Study the drawing (mm; zero at the part's minimum x, y, z) and answer. A direction names the side the tool comes from. Coordinates: 2 decimals unless noted, no trailing zeros. Order: outer loops, then holes, each group sorted by start corner. A loop starts at its lowest first (then second) coordinate and runs counter-clockwise, first axis right, second up. Notation, with made-up numbers: M 76.25,-11 L 121.25,-11 A24 cw 121.25,7 Z; hole C 48.25,42 d11. An arc over 180 degrees is marked long. Use a Markdown table: item, result. Add a question column.
1) Find section B-B on z = 51.5. Write down the section's boundary in (x, y).
2) Find section A-A on y = 12. Write down the section's boundary in (x, z).
3) Find section D-D on x = 88. Write down the section's boundary in (y, z), plus the area to 3 significant figures.
4) The mould has two halves that part along Y. Classify the marked faces 3, 4 and 5: released by +Y, released by -Y, zero draft, split by the parting line, or undercut.
5) Find section C-C on x = 17. Write down the section's boundary in (y, z).
6) Each of these flat-tipped pins is pushed along its axis until it touches: pin 1 Ø2.5 at (x, y) = (66, 45.5) entering from +Z; pin 2 Ø12.5 at (x, y) = (75, 20.5) entering from +Z; pin 3 Ø3.5 at (x, y) = (77.5, 2) entering from +Z. Where does it stop, or does it pass through?
7) Find the intervals of material crossed by probe 1 along Y at (x, z) = (119, 72); probe 2 along X at (y, z) = (34, 51.5); probe 3 along Y at (x, z) = (10, 19), in increasing order. Write a range as [from, to].
8) For the marked faces 1 and 2, determine the directions among +Z, -Z, +X, -X, +Y, -Y from which every point of the face is accessible in a straight line to the end or side of a thin tool.
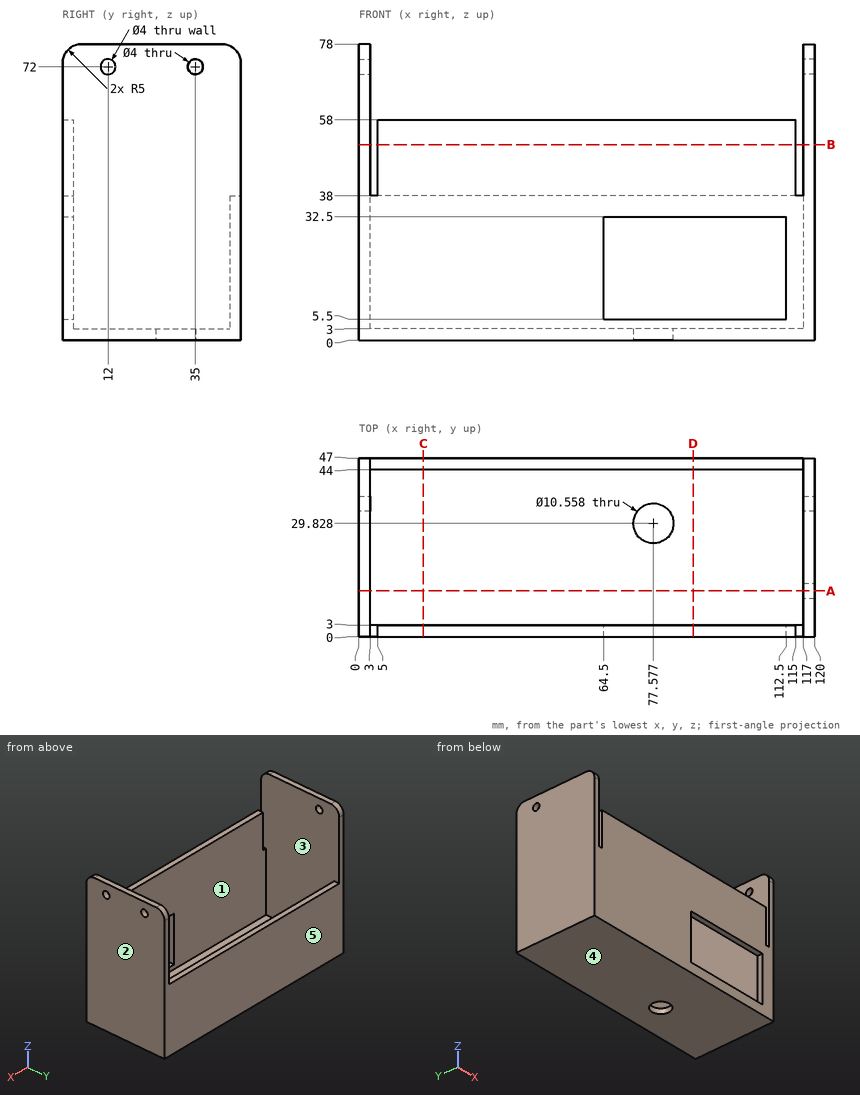
Check result:
| question | item | result |
|---|---|---|
| 1 | outline | M 0,0 L 3,0 L 3,47 L 0,47 Z; M 5,0 L 115,0 L 115,3 L 5,3 Z; M 117,0 L 120,0 L 120,47 L 117,47 Z |
| 2 | outline | M 0,0 L 120,0 L 120,70 L 117,70 L 117,3 L 3,3 L 3,78 L 0,78 Z; M 117,74 L 120,74 L 120,78 L 117,78 Z |
| 3 | outline | M 0,0 L 47,0 L 47,38 L 44,38 L 44,3 L 3,3 L 3,5.5 L 0,5.5 Z; M 0,32.5 L 3,32.5 L 3,58 L 0,58 Z |
| 3 | area | 330 mm2 |
| 4 | face 3 | undercut |
| 4 | face 4 | zero draft |
| 4 | face 5 | released by +Y |
| 5 | outline | M 0,0 L 47,0 L 47,38 L 44,38 L 44,3 L 3,3 L 3,58 L 0,58 Z |
| 6 | pin 1 | stops at z = 38 |
| 6 | pin 2 | stops at z = 3 |
| 6 | pin 3 | stops at z = 58 |
| 7 | probe 1 | y = [0, 10], [14, 33], [37, 47] |
| 7 | probe 2 | x = [0, 3], [117, 120] |
| 7 | probe 3 | y = [0, 3], [44, 47] |
| 8 | face 1 | +Z |
| 8 | face 2 | +Z, -Z, +X, +Y, -Y |
